Input: part model. Units: mm. Frame: model coordinates. A direction names the side the tool comes from. Give positions to 0.01 mm unless a question says otherwise; leave off trailing zeros. Write each loop counter-clockwise with the first axis right and the second up, starting at its lowest first coordinate (ties: lowest second). Pieces come first, ordered by that corner, then holes. Notation, with made-up numbers: (8, -14) -> (31, -14) arc R23 cw to (31, 8) -> close; hole circle Ø6 at (-9.5, -33.75). An arc over 180 degrees is marked (long way). Return JSON: item names as keys, results as strings. Group by question number.
Item 1: Mould query, pull axis X, two halves, no side actions, for faces 1 (the face through (-0.238, 15.926, 5.708)), 2 (the face through (6, 2, 0)). Classes: released by +X, released by -X, zero draft, split by the parting line, or undercut.
Item 2: Set-up query: faces 3 (the face through (0, 12, -6.3)), 4 (the face through (-6, 2, 0)), 5 (the face through (1.532, 1.713, 4.864)), 6 (the face through (0, 12, 6.3)). Return all of +Z, -Z, +X, -X, +Y, -Y with unobstructed straight access to the full face (end or side cutting, diameter ignored); none if empty.
Item 3: Section A-A, the plane y = 13.5. Return loops of the section in (x, z).
Item 4: Pin query (flat end, axial travel): P1, Ø5, axis at x = 5.5, y = 5.5, coming from the -Z side; P2, Ø4, axis at x = -2, y = 6.5, coming from the -Z side; P3, Ø1.8, axis at x = 0, y = 10, coming from the -Z side; P4, Ø5, axis at y = 3.5, z = -2.5, coming from the -X side. Return the tip coordinate at first contact, or that it passes through.
Item 5: Line query: line 1 (Y direction, x = 0, z = 5.55); line 2 (Z direction, x = 1.25, y = 20); line 3 (Y direction, x = 0, z = -6). Output: solid intervals per line, ascending. Write a range as [from, to].
Item 6: Section C-C, the plane y = 10. Return loops of the section in (x, z), then the cut area to 3 significant figures.
Item 7: Section B-B, the plane z = 0. Return loops of the section in (x, y).
from build123d import *

# Parameters (mm, degrees)
SKETCH_1_R          = 6.75
SKETCH_1_R_2        = 4.5
EXTRUDE_1_DEPTH     = 2
SKETCH_2_R          = 5.1000000000000005
CUT_EXTRUDE_1_DEPTH = 1
EXTRUDE_2_DEPTH     = 20
SKETCH_4_R          = 1.1
CUT_EXTRUDE_2_DEPTH = 20
CHAMFER_1_SIZE      = 1
CHAMFER_2_SIZE      = 1
CHAMFER_3_SIZE      = 0.8


with BuildPart() as part:
    # 草图1 → 凸台-拉伸1 (new body)
    with BuildSketch(Plane(origin=(0, 0, 0), x_dir=(1, 0, 0), z_dir=(0, 1, 0))):
        with Locations(Location((0, 0, 0), (0, 0, 270))):
            Circle(SKETCH_1_R)
        with Locations(Location((0, 0, 0), (0, 0, 270))):
            Circle(SKETCH_1_R_2, mode=Mode.SUBTRACT)
    extrude(amount=EXTRUDE_1_DEPTH)

    # 草图2 → 切除-拉伸1 (cut)
    with BuildSketch(Plane(origin=(0, 2, 0), x_dir=(1, 0, 0), z_dir=(0, 1, 0))):
        with Locations(Location((0, 0, 0), (0, 0, 270))):
            Circle(SKETCH_2_R)
    extrude(amount=-CUT_EXTRUDE_1_DEPTH, mode=Mode.SUBTRACT)

    # 草图3 → 凸台-拉伸2 (add)
    with BuildSketch(Plane(origin=(0, 2, 0), x_dir=(1, 0, 0), z_dir=(0, 1, 0))):
        with BuildLine():
            ThreePointArc((-2.4233241632105296, 6.299999999999999), (-3.4747665686142524, 5.786924683598426), (-4.421820891895102, 5.1))
            Line((-4.421820891895103, 5.1), (4.421820891895103, 5.1))
            ThreePointArc((4.421820891895103, 5.099999999999999), (3.4747665686142533, 5.786924683598425), (2.4233241632105287, 6.299999999999999))
            Line((2.4233241632105287, 6.299999999999999), (-2.4233241632105287, 6.299999999999999))
        make_face()
        with BuildLine():
            Line((4.421820891895103, -5.1), (-4.421820891895103, -5.1))
            ThreePointArc((-4.421820891895104, -5.099999999999999), (-3.4747665686142537, -5.786924683598424), (-2.4233241632105327, -6.299999999999998))
            Line((-2.4233241632105287, -6.299999999999999), (2.4233241632105287, -6.299999999999999))
            ThreePointArc((2.4233241632105305, -6.299999999999999), (3.4747665686142515, -5.786924683598426), (4.4218208918951, -5.100000000000002))
        make_face()
    extrude(amount=EXTRUDE_2_DEPTH)

    # 草图4 → 切除-拉伸2 (cut)
    with BuildSketch(Plane.XY.offset(6.299999999999999)):
        with Locations((0, 17)):
            Circle(SKETCH_4_R)
        with Locations((0, 10)):
            Circle(SKETCH_4_R)
    extrude(amount=-CUT_EXTRUDE_2_DEPTH, mode=Mode.SUBTRACT)

    # 倒角1
    chamfer_1_edges = [part.edges().sort_by_distance(p)[0] for p in [
        (2.07e-15, 0, -6.75),
    ]]
    chamfer(chamfer_1_edges, length=CHAMFER_1_SIZE)

    # 倒角2
    # the kernel refuses this chamfer: 1 mm, written as the material it adds along each edge
    with BuildSketch(Plane(origin=(-4.99500715117644, 2, 6.299999999999999), x_dir=(0, -0.02749587661058627, 0.9996219169112968), z_dir=(1, 0, 0))) as chamfer_2_piece_1_section:
        Polygon((CHAMFER_2_SIZE * 0.999621916911, -CHAMFER_2_SIZE * 0.0274958766106), (-CHAMFER_2_SIZE * 0.0274958766106, -CHAMFER_2_SIZE * 0.999621916911), (0, 0), align=None)
    chamfer_2_piece_1 = extrude(amount=9.99001430235288, mode=Mode.PRIVATE)
    chamfer_2_piece_1 = chamfer_2_piece_1 & Plane(origin=(0, 2.4270240962086875, 0), x_dir=(-1.8e-16, 0, 1), z_dir=(0, -1, 0)) * Cylinder(6.75, 24, mode=Mode.PRIVATE)
    add(chamfer_2_piece_1)
    with BuildSketch(Plane(origin=(4.99500715117644, 2, -6.299999999999999), x_dir=(0, -0.02749587661058627, -0.9996219169112968), z_dir=(-1, 0, 0))) as chamfer_2_piece_2_section:
        Polygon((CHAMFER_2_SIZE * 0.999621916911, -CHAMFER_2_SIZE * 0.0274958766106), (-CHAMFER_2_SIZE * 0.0274958766106, -CHAMFER_2_SIZE * 0.999621916911), (0, 0), align=None)
    chamfer_2_piece_2 = extrude(amount=9.99001430235288, mode=Mode.PRIVATE)
    chamfer_2_piece_2 = chamfer_2_piece_2 & Plane(origin=(0, 2.4270241038722706, 0), x_dir=(-1.8e-16, 0, 1), z_dir=(0, -1, 0)) * Cylinder(6.75, 24, mode=Mode.PRIVATE)
    add(chamfer_2_piece_2)

    # 倒角3
    # the kernel refuses this chamfer: 0.8 mm, written as the material it adds along each edge
    with BuildSketch(Plane(origin=(6.22e-15, 2, -5.1), x_dir=(0, 0.9996219169112968, -0.027495876610586285), z_dir=(1, 0, 0))) as chamfer_3_piece_1_section:
        Polygon((CHAMFER_3_SIZE * 0.999621916911, CHAMFER_3_SIZE * 0.0274958766106), (-CHAMFER_3_SIZE * 0.0274958766106, CHAMFER_3_SIZE * 0.999621916911), (0, 0), align=None)
    chamfer_3_piece_1 = extrude(amount=6.479167282267824, mode=Mode.PRIVATE)
    chamfer_3_piece_1 = chamfer_3_piece_1 & Plane(origin=(0, 2.278466401916116, 0), x_dir=(-1.8e-16, 0, 1), z_dir=(0, -1, 0)) * Cylinder(6.75, 17, mode=Mode.PRIVATE)
    chamfer_3_piece_1 = chamfer_3_piece_1 - Plane(origin=(0, 2.278466401916116, 0), x_dir=(-1.8e-16, 0, 1), z_dir=(0, 1, 0)) * Cylinder(5.1000000000000005, 17, mode=Mode.PRIVATE)
    add(chamfer_3_piece_1)
    with BuildSketch(Plane(origin=(-6.479167282267831, 2, -5.1), x_dir=(0, 0.9996219169112968, -0.027495876610586285), z_dir=(1, 0, 0))) as chamfer_3_piece_2_section:
        Polygon((CHAMFER_3_SIZE * 0.999621916911, CHAMFER_3_SIZE * 0.0274958766106), (-CHAMFER_3_SIZE * 0.0274958766106, CHAMFER_3_SIZE * 0.999621916911), (0, 0), align=None)
    chamfer_3_piece_2 = extrude(amount=6.479167282267837, mode=Mode.PRIVATE)
    chamfer_3_piece_2 = chamfer_3_piece_2 & Plane(origin=(0, 2.27846640235757, 0), x_dir=(-1.8e-16, 0, 1), z_dir=(0, -1, 0)) * Cylinder(6.75, 17, mode=Mode.PRIVATE)
    chamfer_3_piece_2 = chamfer_3_piece_2 - Plane(origin=(0, 2.27846640235757, 0), x_dir=(-1.8e-16, 0, 1), z_dir=(0, 1, 0)) * Cylinder(5.1000000000000005, 17, mode=Mode.PRIVATE)
    add(chamfer_3_piece_2)
    with BuildSketch(Plane(origin=(-8.9e-16, 2, 5.1), x_dir=(0, -0.027495876610586285, -0.9996219169112968), z_dir=(-1, 0, 0))) as chamfer_3_piece_3_section:
        Polygon((CHAMFER_3_SIZE * 0.999621916911, -CHAMFER_3_SIZE * 0.0274958766106), (-CHAMFER_3_SIZE * 0.0274958766106, -CHAMFER_3_SIZE * 0.999621916911), (0, 0), align=None)
    chamfer_3_piece_3 = extrude(amount=6.479167282267829, mode=Mode.PRIVATE)
    chamfer_3_piece_3 = chamfer_3_piece_3 & Plane(origin=(0, 2.2784664022483097, 0), x_dir=(-1.8e-16, 0, 1), z_dir=(0, -1, 0)) * Cylinder(6.75, 17, mode=Mode.PRIVATE)
    chamfer_3_piece_3 = chamfer_3_piece_3 - Plane(origin=(0, 2.2784664022483097, 0), x_dir=(-1.8e-16, 0, 1), z_dir=(0, 1, 0)) * Cylinder(5.1000000000000005, 17, mode=Mode.PRIVATE)
    add(chamfer_3_piece_3)
    with BuildSketch(Plane(origin=(6.479167282267831, 2, 5.1), x_dir=(0, -0.027495876610586285, -0.9996219169112968), z_dir=(-1, 0, 0))) as chamfer_3_piece_4_section:
        Polygon((CHAMFER_3_SIZE * 0.999621916911, -CHAMFER_3_SIZE * 0.0274958766106), (-CHAMFER_3_SIZE * 0.0274958766106, -CHAMFER_3_SIZE * 0.999621916911), (0, 0), align=None)
    chamfer_3_piece_4 = extrude(amount=6.479167282267832, mode=Mode.PRIVATE)
    chamfer_3_piece_4 = chamfer_3_piece_4 & Plane(origin=(0, 2.278466402305348, 0), x_dir=(-1.8e-16, 0, 1), z_dir=(0, -1, 0)) * Cylinder(6.75, 17, mode=Mode.PRIVATE)
    chamfer_3_piece_4 = chamfer_3_piece_4 - Plane(origin=(0, 2.278466402305348, 0), x_dir=(-1.8e-16, 0, 1), z_dir=(0, 1, 0)) * Cylinder(5.1000000000000005, 17, mode=Mode.PRIVATE)
    add(chamfer_3_piece_4)


solid = part.part
Answer below:
{
 "1": {"face 1": "undercut", "face 2": "zero draft"},
 "2": {"face 3": "-Z, +X, -X, +Y", "face 4": "+X, -X, +Y", "face 5": "+Y", "face 6": "+Z, +X, -X, +Y"},
 "3": {"outline": "(-4.42, -5.1) arc R6.75 ccw to (-2.42, -6.3) -> (2.42, -6.3) arc R6.75 ccw to (4.42, -5.1) -> close; (-4.42, 5.1) -> (4.42, 5.1) arc R6.75 ccw to (2.42, 6.3) -> (-2.42, 6.3) arc R6.75 ccw to start"},
 "4": {"P1": "stops at z = -6.05", "P2": "stops at z = -6.3", "P3": "passes through", "P4": "stops at x = -6.73"},
 "5": {"line 1": "y = [0, 8.9], [11.1, 15.9], [18.1, 22]", "line 2": "z = [-6.3, -5.1], [5.1, 6.3]", "line 3": "y = [0.25, 8.9], [11.1, 15.9], [18.1, 22]"},
 "6": {"outline": "(-4.42, -5.1) arc R6.75 ccw to (-2.42, -6.3) -> (-1.1, -6.3) -> (-1.1, -5.1) -> close; (-4.42, 5.1) -> (-1.1, 5.1) -> (-1.1, 6.3) -> (-2.42, 6.3) arc R6.75 ccw to start; (1.1, -6.3) -> (2.42, -6.3) arc R6.75 ccw to (4.42, -5.1) -> (1.1, -5.1) -> close; (1.1, 5.1) -> (4.42, 5.1) arc R6.75 ccw to (2.42, 6.3) -> (1.1, 6.3) -> close", "area": "11.8 mm2"},
 "7": {"outline": "(-6.75, 1) -> (-5.75, 0) -> (-4.5, 0) -> (-4.5, 1) -> (-5.1, 1) -> (-5.1, 2) -> (-6.75, 2) -> close; (4.5, 0) -> (5.75, 0) -> (6.75, 1) -> (6.75, 2) -> (5.1, 2) -> (5.1, 1) -> (4.5, 1) -> close"}
}
